Read the model definition and answer for the solid it produces. Units are mm, in the model's axes. Round coordinates to 2 decimals unless told otherwise and drop trailing zeros. Order: outer loops, then holes, each group sorted by start corner. A loop starts at its lowest first (then second) coordinate and runs counter-clockwise, first axis right, second up.
from build123d import *

# Parameters (mm, degrees)
SKETCH_W                     = 15.24
SKETCH_H                     = 5.08
PAD_DEPTH                    = 1.6
SKETCH001_R                  = 0.51
POCKET_DEPTH                 = 33.888707
SKETCH001_LINEARPATTERN_2_R  = 0.51
POCKET_LINEARPATTERN_2_DEPTH = 33.888707
SKETCH001_LINEARPATTERN_3_R  = 0.51
POCKET_LINEARPATTERN_3_DEPTH = 33.888707
SKETCH001_LINEARPATTERN_4_R  = 0.51
POCKET_LINEARPATTERN_4_DEPTH = 33.888707
SKETCH001_LINEARPATTERN_5_R  = 0.51
POCKET_LINEARPATTERN_5_DEPTH = 33.888707
SKETCH001_LINEARPATTERN_6_R  = 0.51
POCKET_LINEARPATTERN_6_DEPTH = 33.888707
SKETCH001_LINEARPATTERN_7_R  = 0.51
POCKET_LINEARPATTERN_7_DEPTH = 33.888707
LINEARPATTERN003_COUNT       = 3
LINEARPATTERN003_PITCH       = 2.54


with BuildPart() as part:
    # Sketch → Pad (new body)
    with BuildSketch(Plane.XY):
        Rectangle(SKETCH_W, SKETCH_H)
    extrude(amount=PAD_DEPTH)

    # Sketch001 → Pocket (cut, through all)
    with BuildSketch(Plane.XY.offset(1.6)):
        with Locations((-7.62, 2.54)):
            Circle(SKETCH001_R)
    pocket = extrude(amount=-POCKET_DEPTH, mode=Mode.SUBTRACT)

    # Sketch001 LinearPattern 2 → Pocket LinearPattern 2 (cut, through all)
    with BuildSketch(Plane(origin=(2.54, 0, 1.6), x_dir=(1, 0, 0), z_dir=(0, 0, 1))):
        with Locations((-7.62, 2.54)):
            Circle(SKETCH001_LINEARPATTERN_2_R)
    pocket_linearpattern_2 = extrude(amount=-POCKET_LINEARPATTERN_2_DEPTH, mode=Mode.SUBTRACT)

    # Sketch001 LinearPattern 3 → Pocket LinearPattern 3 (cut, through all)
    with BuildSketch(Plane(origin=(5.08, 0, 1.6), x_dir=(1, 0, 0), z_dir=(0, 0, 1))):
        with Locations((-7.62, 2.54)):
            Circle(SKETCH001_LINEARPATTERN_3_R)
    pocket_linearpattern_3 = extrude(amount=-POCKET_LINEARPATTERN_3_DEPTH, mode=Mode.SUBTRACT)

    # Sketch001 LinearPattern 4 → Pocket LinearPattern 4 (cut, through all)
    with BuildSketch(Plane(origin=(7.62, 0, 1.6), x_dir=(1, 0, 0), z_dir=(0, 0, 1))):
        with Locations((-7.62, 2.54)):
            Circle(SKETCH001_LINEARPATTERN_4_R)
    pocket_linearpattern_4 = extrude(amount=-POCKET_LINEARPATTERN_4_DEPTH, mode=Mode.SUBTRACT)

    # Sketch001 LinearPattern 5 → Pocket LinearPattern 5 (cut, through all)
    with BuildSketch(Plane(origin=(10.16, 0, 1.6), x_dir=(1, 0, 0), z_dir=(0, 0, 1))):
        with Locations((-7.62, 2.54)):
            Circle(SKETCH001_LINEARPATTERN_5_R)
    pocket_linearpattern_5 = extrude(amount=-POCKET_LINEARPATTERN_5_DEPTH, mode=Mode.SUBTRACT)

    # Sketch001 LinearPattern 6 → Pocket LinearPattern 6 (cut, through all)
    with BuildSketch(Plane(origin=(12.7, 0, 1.6), x_dir=(1, 0, 0), z_dir=(0, 0, 1))):
        with Locations((-7.62, 2.54)):
            Circle(SKETCH001_LINEARPATTERN_6_R)
    pocket_linearpattern_6 = extrude(amount=-POCKET_LINEARPATTERN_6_DEPTH, mode=Mode.SUBTRACT)

    # Sketch001 LinearPattern 7 → Pocket LinearPattern 7 (cut, through all)
    with BuildSketch(Plane(origin=(15.24, 0, 1.6), x_dir=(1, 0, 0), z_dir=(0, 0, 1))):
        with Locations((-7.62, 2.54)):
            Circle(SKETCH001_LINEARPATTERN_7_R)
    pocket_linearpattern_7 = extrude(amount=-POCKET_LINEARPATTERN_7_DEPTH, mode=Mode.SUBTRACT)

    # LinearPattern003: Pocket, Pocket LinearPattern 2, Pocket LinearPattern 3, Pocket LinearPattern 4, Pocket LinearPattern 5, Pocket LinearPattern 6, Pocket LinearPattern 7 ×3
    with Locations(*[(0, -i * LINEARPATTERN003_PITCH, 0) for i in range(1, LINEARPATTERN003_COUNT)]):
        add(pocket, mode=Mode.SUBTRACT)
        add(pocket_linearpattern_2, mode=Mode.SUBTRACT)
        add(pocket_linearpattern_3, mode=Mode.SUBTRACT)
        add(pocket_linearpattern_4, mode=Mode.SUBTRACT)
        add(pocket_linearpattern_5, mode=Mode.SUBTRACT)
        add(pocket_linearpattern_6, mode=Mode.SUBTRACT)
        add(pocket_linearpattern_7, mode=Mode.SUBTRACT)


solid = part.part
Q1. A cutting plane is placed at D-D, the plane z = 0.85. Give the number of separate pieces and of enclosed holes in the cut face, plus the area to 3 significant figures.
Outcome:
separate pieces: 1
enclosed holes: 5
area: 67.6 mm2
Q2. Straight lines are drawn through the part: probe 1 along X at (y, z) = (-0.05, 0.8); probe 2 along Y at (x, z) = (0, 1.35); probe 3 along Y at (x, z) = (4.75, 1.05). For each, find the intervals that lie inside material, in ascending order.
Outcome:
probe 1: x = -7.11 to -5.59, -4.57 to -3.05, -2.03 to -0.51, 0.51 to 2.03, 3.05 to 4.57, 5.59 to 7.11
probe 2: y = -2.03 to -0.51, 0.51 to 2.03
probe 3: y = -2.15 to -0.39, 0.39 to 2.15
Q3. A cutting plane is placed at A-A, the plane x = 0. Give the vertices of the cut face in (y, z).
Outcome:
outline: (-2.03, 0) - (-0.51, 0) - (-0.51, 1.6) - (-2.03, 1.6) - close; (0.51, 0) - (2.03, 0) - (2.03, 1.6) - (0.51, 1.6) - close
Q4. A cutting plane is placed at B-B, the plane y = 0. Give the vertices of the cut face in (x, z).
Outcome:
outline: (-7.11, 0) - (-5.59, 0) - (-5.59, 1.6) - (-7.11, 1.6) - close; (-4.57, 0) - (-3.05, 0) - (-3.05, 1.6) - (-4.57, 1.6) - close; (-2.03, 0) - (-0.51, 0) - (-0.51, 1.6) - (-2.03, 1.6) - close; (0.51, 0) - (2.03, 0) - (2.03, 1.6) - (0.51, 1.6) - close; (3.05, 0) - (4.57, 0) - (4.57, 1.6) - (3.05, 1.6) - close; (5.59, 0) - (7.11, 0) - (7.11, 1.6) - (5.59, 1.6) - close
Q5. A cutting plane is placed at C-C, the plane x = -4.75. Give the vertices of the cut face in (y, z).
Outcome:
outline: (-2.15, 0) - (-0.39, 0) - (-0.39, 1.6) - (-2.15, 1.6) - close; (0.39, 0) - (2.15, 0) - (2.15, 1.6) - (0.39, 1.6) - close
Q6. For a pull along Y with two mould halves and no side action, classify faces 1 (the face through (-2.07, -0.2, 0.81)), 2 (the face through (-0.01, 2.03, 0.81)), 3 (the face through (-7.62, 1, 1)) as released by +Y, released by -Y, zero draft, split by the parting line, or undercut.
Outcome:
face 1: undercut
face 2: released by +Y
face 3: zero draft
Q7. Flat-ended cylindrical pins translate along their axes: pin 1 (1.2 mm diameter, centred on x = -5.08, y = 0, fed in from +Z); pin 2 (0.9 mm diameter, centred on x = -2.54, y = 0, fed in from -Z). Find the tip coordinate at first contact, or state that the pin passes through.
Outcome:
pin 1: stops at z = 1.6
pin 2: passes through
